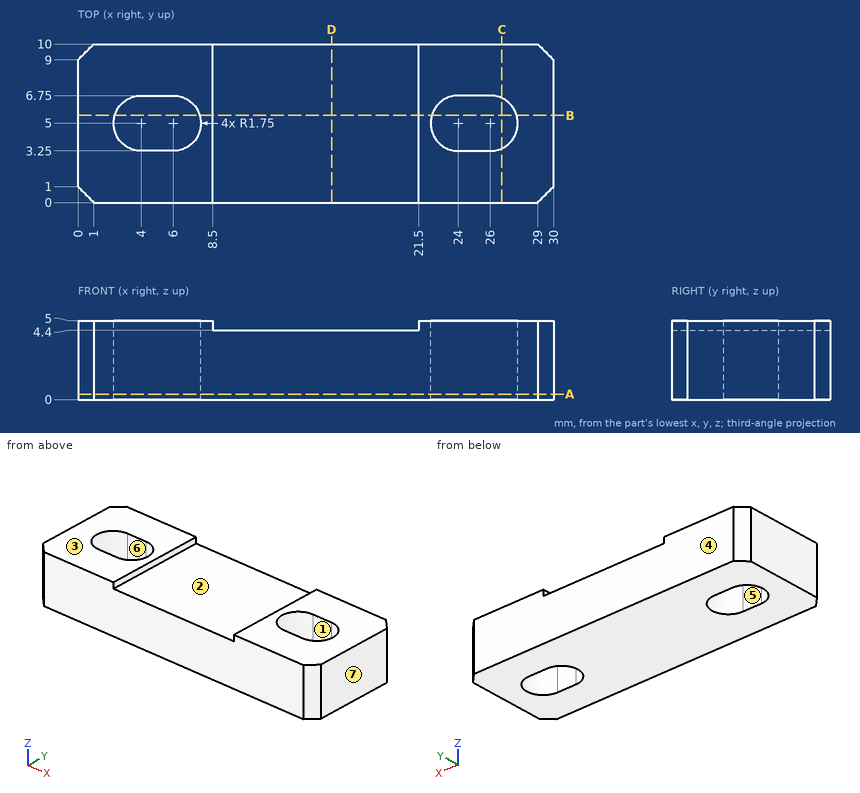
Verification items for this drawing (mm, ordinates from the low corner). A direction names the side the tool comes from. Give positions to 0.01 mm unless a question says otherwise; leave off trailing zeros. Loops run counter-clockwise (first coordinate to the right, second up) from the corner with the lowest first, then second, coordinate; pieces in that order, holes last.
1. Cross-section at B-B on y = 5.5. Record the cut outline in (x, z).
Derived:
outline: (0, 0) - (2.32, 0) - (2.32, 5) - (0, 5) - close; (7.68, 0) - (22.32, 0) - (22.32, 5) - (21.5, 5) - (21.5, 4.4) - (8.5, 4.4) - (8.5, 5) - (7.68, 5) - close; (27.68, 0) - (30, 0) - (30, 5) - (27.68, 5) - close
2. Cross-section at C-C on x = 26.75. Record the cut outline in (y, z).
Derived:
outline: (0, 0) - (3.42, 0) - (3.42, 5) - (0, 5) - close; (6.58, 0) - (10, 0) - (10, 5) - (6.58, 5) - close
3. Release check for a two-part mould opening along Y. For the marked faces 4, 5, 6 and 7 record: +Y half, -Y half, draft (parallel to the pull), parting line (faces both ways), or undercut.
Derived:
face 4: +Y half
face 5: undercut
face 6: undercut
face 7: draft
4. Material ranges on probe 1 along X at (y, z) = (3.75, 4.7); probe 2 along X at (y, z) = (4.75, 0.8); probe 3 along Y at (x, z) = (26, 2.05), recorded low to high.
Derived:
probe 1: x = 0 to 2.78, 7.22 to 8.5, 21.5 to 22.78, 27.22 to 30
probe 2: x = 0 to 2.27, 7.73 to 22.27, 27.73 to 30
probe 3: y = 0 to 3.25, 6.75 to 10
5. Cross-section at A-A on z = 0.35. Record the cut outline in (x, y), and give its area (3 significant figures).
Derived:
outline: (0, 1) - (1, 0) - (29, 0) - (30, 1) - (30, 9) - (29, 10) - (1, 10) - (0, 9) - close; hole (4, 3.25) - (6, 3.25) arc R1.75 ccw to (6, 6.75) - (4, 6.75) arc R1.75 ccw to start; hole (24, 3.25) - (26, 3.25) arc R1.75 ccw to (26, 6.75) - (24, 6.75) arc R1.75 ccw to start
area: 265 mm2
6. Go/stop test with a flat-tipped pin: P1, Ø4, axis at x = 23, y = 3.5, coming from the -Z side. Record where the tip stops, or that it passes through.
Derived:
P1: stops at z = 0
7. Cross-section at D-D on x = 16. Record the cut outline in (y, z), and give its area (3 significant figures).
Derived:
outline: (0, 0) - (10, 0) - (10, 4.4) - (0, 4.4) - close
area: 44.0 mm2
8. Tool access check on the marked faces 1, 2 and 3. Record the directions out of +Z, -Z, +X, -X, +Y, -Y that give a thin tool (end or side, any length) a straight path to the whole face; none if there is none.
Derived:
face 1: +Z, -Z
face 2: +Z, +Y, -Y
face 3: +Z, +X, -X, +Y, -Y
